Could you check a few things on this model? Use its own coordinates, in mm. A direction names the side the tool comes from. Round coordinates to 2 decimals unless told otherwise and drop trailing zeros. Order: outer loops, then holes, each group sorted by start corner. A loop starts at its lowest first (then second) coordinate and runs counter-clockwise, first axis right, second up. Notation, with made-up numbers: (39.25, -7.75) -> (52.25, -7.75) arc R11 ccw to (52.25, 9.25) -> close; hole circle Ø6 at (48.5, 9). An arc over 180 degrees is marked (long way). One line per question, with ' | ' between items.
```python
from build123d import *

# Parameters (mm, degrees)
BOSS_EXTRUDE1_DEPTH = 145.01147666
SKETCH2_W           = 9.451272727
SKETCH2_H           = 145.01147666
BOSS_EXTRUDE2_DEPTH = 30
SKETCH3_W           = 9.451272727
SKETCH3_H           = 30
BOSS_EXTRUDE3_DEPTH = 284.3485
SKETCH5_W           = 10
SKETCH5_H           = 60
CUT_EXTRUDE1_DEPTH  = 240
SKETCH6_W           = 5
SKETCH6_H           = 20
CUT_EXTRUDE2_DEPTH  = 472.121269354
FILLET1_R           = 10
FILLET2_R           = 10
FILLET3_R           = 10
SKETCH8_W           = 5
SKETCH8_H           = 20
CUT_EXTRUDE3_DEPTH  = 472.121269409
BOSS_EXTRUDE4_DEPTH = 30.8583
FILLET4_R           = 5
SKETCH10_R          = 1.0922
CUT_EXTRUDE4_DEPTH  = 5


with BuildPart() as part:
    # Sketch1 → Boss-Extrude1 (new body)
    with BuildSketch(Plane(origin=(0, 0, 0), x_dir=(1, 0, 0), z_dir=(0, 1, 0))):
        with BuildLine():
            Line((-77.272727273, 0), (-86.724, 0))
            ThreePointArc((-86.724, 0), (0, 86.724), (86.724, 0))
            Line((86.724, 0), (77.272727273, 0))
            ThreePointArc((77.272727273, 0), (0, 77.272727273), (-77.272727273, 0))
        make_face()
    extrude(amount=BOSS_EXTRUDE1_DEPTH)

    # Sketch2 → Boss-Extrude2 (add)
    with BuildSketch(Plane.XY):
        with Locations((81.998363637, 72.50573833)):
            Rectangle(SKETCH2_W, SKETCH2_H)
        with Locations((-81.998363637, 72.50573833)):
            Rectangle(SKETCH2_W, SKETCH2_H)
    extrude(amount=BOSS_EXTRUDE2_DEPTH)

    # Sketch3 → Boss-Extrude3 (add)
    with BuildSketch(Plane(origin=(0, 145.01147666, 0), x_dir=(1, 0, 0), z_dir=(0, 1, 0))):
        with Locations((-81.998363637, -15)):
            Rectangle(SKETCH3_W, SKETCH3_H)
        with Locations((81.998363637, -15)):
            Rectangle(SKETCH3_W, SKETCH3_H)
    extrude(amount=BOSS_EXTRUDE3_DEPTH)

    # Sketch5 → Cut-Extrude1 (cut)
    with BuildSketch(Plane.ZY.offset(86.724)):
        with Locations((10, 389.35997666)):
            Rectangle(SKETCH5_W, SKETCH5_H)
    extrude(amount=-CUT_EXTRUDE1_DEPTH, mode=Mode.SUBTRACT)

    # Sketch6 → Cut-Extrude2 (cut, through all)
    with BuildSketch(Plane.ZY.offset(86.724)):
        with Locations((22.5, 389.35997666)):
            Rectangle(SKETCH6_W, SKETCH6_H)
    extrude(amount=-CUT_EXTRUDE2_DEPTH, mode=Mode.SUBTRACT)

    # Fillet1
    fillet1_edges = [part.edges().sort_by_distance(p)[0] for p in [
        (-81.998363636, 429.35997666, 0),
        (-81.998363636, 429.35997666, 30),
        (81.998363636, 429.35997666, 0),
        (81.998363636, 429.35997666, 30),
    ]]
    fillet(fillet1_edges, radius=FILLET1_R)

    # Fillet2
    fillet2_edges = [part.edges().sort_by_distance(p)[0] for p in [
        (81.998363636, 0, 30),
        (-81.998363636, 0, 30),
    ]]
    fillet(fillet2_edges, radius=FILLET2_R)

    # Fillet3
    # the kernel refuses this fillet: 10 mm, written as the material it adds along each edge
    with BuildSketch(Plane(origin=(-111.724, 145.01147666, 0), x_dir=(0, 1, 0), z_dir=(1, 0, 0))) as fillet3_piece_1_section:
        with BuildLine():
            CenterArc((FILLET3_R, -FILLET3_R), FILLET3_R, 90, 90)
            Line((0, -FILLET3_R), (0, 0))
            Line((0, 0), (FILLET3_R, 0))
        make_face()
    fillet3_piece_1 = extrude(amount=59.451272727, mode=Mode.PRIVATE)
    fillet3_piece_1 = fillet3_piece_1 & Plane(origin=(0, 147.252284307, 0), x_dir=(-1, 0, 0), z_dir=(0, -1, 0)) * Cylinder(86.724, 159, mode=Mode.PRIVATE)
    fillet3_piece_1 = fillet3_piece_1 - Plane(origin=(0, 147.252284307, 0), x_dir=(1, 0, 0), z_dir=(0, -1, 0)) * Cylinder(77.272727273, 159, mode=Mode.PRIVATE)
    add(fillet3_piece_1)
    with BuildSketch(Plane(origin=(52.272727273, 145.01147666, 0), x_dir=(0, 0, -1), z_dir=(1, 0, 0))) as fillet3_piece_2_section:
        with BuildLine():
            CenterArc((FILLET3_R, FILLET3_R), FILLET3_R, 180, 90)
            Line((0, FILLET3_R), (0, 0))
            Line((0, 0), (FILLET3_R, 0))
        make_face()
    fillet3_piece_2 = extrude(amount=59.451272727, mode=Mode.PRIVATE)
    fillet3_piece_2 = fillet3_piece_2 & Plane(origin=(0, 145.87973925, 0), x_dir=(-1, 0, 0), z_dir=(0, -1, 0)) * Cylinder(86.724, 159, mode=Mode.PRIVATE)
    fillet3_piece_2 = fillet3_piece_2 - Plane(origin=(0, 145.87973925, 0), x_dir=(1, 0, 0), z_dir=(0, -1, 0)) * Cylinder(77.272727273, 159, mode=Mode.PRIVATE)
    add(fillet3_piece_2)

    # Sketch8 → Cut-Extrude3 (cut, through all)
    with BuildSketch(Plane.ZY.offset(86.724)):
        with Locations((22.5, 40)):
            Rectangle(SKETCH8_W, SKETCH8_H)
    extrude(amount=-CUT_EXTRUDE3_DEPTH, mode=Mode.SUBTRACT)

    # Sketch9 → Boss-Extrude4 (add, symmetric)
    with BuildSketch(Plane(origin=(0, 80.01147666, 0), x_dir=(1, 0, 0), z_dir=(0, 1, 0))):
        with BuildLine():
            Line((-26.79918982, 92.479425319), (-26.79918982, 82.479425319))
            ThreePointArc((-26.79918982, 82.479425319), (0, 86.724), (26.79918982, 82.479425319))
            Line((26.79918982, 82.479425319), (26.79918982, 92.479425319))
            Line((26.79918982, 92.479425319), (-26.79918982, 92.479425319))
        make_face()
    extrude(amount=BOSS_EXTRUDE4_DEPTH, both=True)

    # Fillet4
    fillet4_edges = [part.edges().sort_by_distance(p)[0] for p in [
        (0, 110.86977666, -92.479425319),
        (26.79918982, 80.01147666, -92.479425319),
        (-26.79918982, 80.01147666, -92.479425319),
        (0, 49.15317666, -92.479425319),
    ]]
    fillet(fillet4_edges, radius=FILLET4_R)

    # Sketch10 → Cut-Extrude4 (cut)
    with BuildSketch(Plane(origin=(0, 0, -92.479425319), x_dir=(-1, 0, 0), z_dir=(0, 0, -1))):
        with Locations((-16.79918982, 100.86977666)):
            Circle(SKETCH10_R)
        with Locations((16.79918982, 100.86977666)):
            Circle(SKETCH10_R)
        with Locations((-16.79918982, 59.15317666)):
            Circle(SKETCH10_R)
        with Locations((16.79918982, 59.15317666)):
            Circle(SKETCH10_R)
    extrude(amount=-CUT_EXTRUDE4_DEPTH, mode=Mode.SUBTRACT)


solid = part.part
```
1. I want a section at C-C on z = -30. List the corners of the cut face in (x, y) for me.
From the geometry:
outline: (-81.37, 0) -> (-71.21, 0) -> (-71.21, 145.01) -> (-81.37, 145.01) -> close; (71.21, 0) -> (81.37, 0) -> (81.37, 145.01) -> (71.21, 145.01) -> close
2. If we mould it in two halves opening along Y, with no side actions, what happens to faces 1 (the face through (77.273, 212, 15)), 2 (the face through (82, 429.36, 15)), 3 (the face through (-26, 0, -73)), 4 (the face through (82, 359.36, 10))? For each: pulls with the +Y half, pulls with the -Y half, needs draft (parallel to the pull), parting line crosses it, or undercut.
From the geometry:
face 1: needs draft | face 2: pulls with the +Y half | face 3: pulls with the -Y half | face 4: undercut
3. I'm going to push flat-ended pins straight in: pin 1 (3 mm diameter, centred on y = 99.5, z = -48.5, fed in from +X); pin 2 (2.5 mm diameter, centred on x = 82, z = 21.5, fed in from +Y); pin 3 (4.5 mm diameter, centred on x = -81, y = 36, fed in from -Z). Where does each tip first touch, or does it pass through?
From the geometry:
pin 1: stops at x = 72.88 | pin 2: stops at y = 429.36 | pin 3: stops at z = -36.32
4. I want a section at B-B on y = 265.5. List the corners of the cut face in (x, z) for me.
From the geometry:
outline: (-86.72, 0) -> (-77.27, 0) -> (-77.27, 30) -> (-86.72, 30) -> close; (77.27, 0) -> (86.72, 0) -> (86.72, 30) -> (77.27, 30) -> close
5. I want a section at D-D on x = 0. List the corners of the cut face in (y, z) for me.
From the geometry:
outline: (0, -86.72) -> (49.15, -86.72) -> (49.15, -87.48) arc R5 ccw to (54.15, -92.48) -> (105.87, -92.48) arc R5 ccw to (110.87, -87.48) -> (110.87, -86.72) -> (145.01, -86.72) -> (145.01, -77.27) -> (0, -77.27) -> close
6. On a 3-axis mill with a long thin cutter (end or side, diameter ignored), from which of +Z, -Z, +X, -X, +Y, -Y can I reach the whole of each face in a straight line? I mean faces 5 (the face through (82, 285, 0)), 6 (the face through (82, 389, 20)), 7 (the face through (-82, 429.36, 15)), 8 (the face through (-77.273, 212, 15)), 9 (the face through (-81.9, 426.5, 27)). Say none if no direction works.
From the geometry:
face 5: -Z, +X, -X, +Y | face 6: +X, -X | face 7: +Z, -Z, +X, -X, +Y | face 8: +Z, +Y, -Y | face 9: +Z, +X, -X, +Y
7. I want a section at A-A on y = 370. List the corners of the cut face in (x, z) for me.
From the geometry:
outline: (-86.72, 0) -> (-77.27, 0) -> (-77.27, 5) -> (-86.72, 5) -> close; (-86.72, 15) -> (-77.27, 15) -> (-77.27, 30) -> (-86.72, 30) -> close; (77.27, 0) -> (86.72, 0) -> (86.72, 5) -> (77.27, 5) -> close; (77.27, 15) -> (86.72, 15) -> (86.72, 30) -> (77.27, 30) -> close
8. I need wall thicknesses on probe 1 along X at (y, z) = (22.5, 20.5); probe 2 along Y at (x, z) = (73.5, -31); probe 3 along X at (y, z) = (72, -11.5). Which ranges of each line are inside material? Lowest first, please.
From the geometry:
probe 1: x = -86.72 to -77.27, 77.27 to 86.72 | probe 2: y = 0 to 145.01 | probe 3: x = -85.96 to -76.41, 76.41 to 85.96
